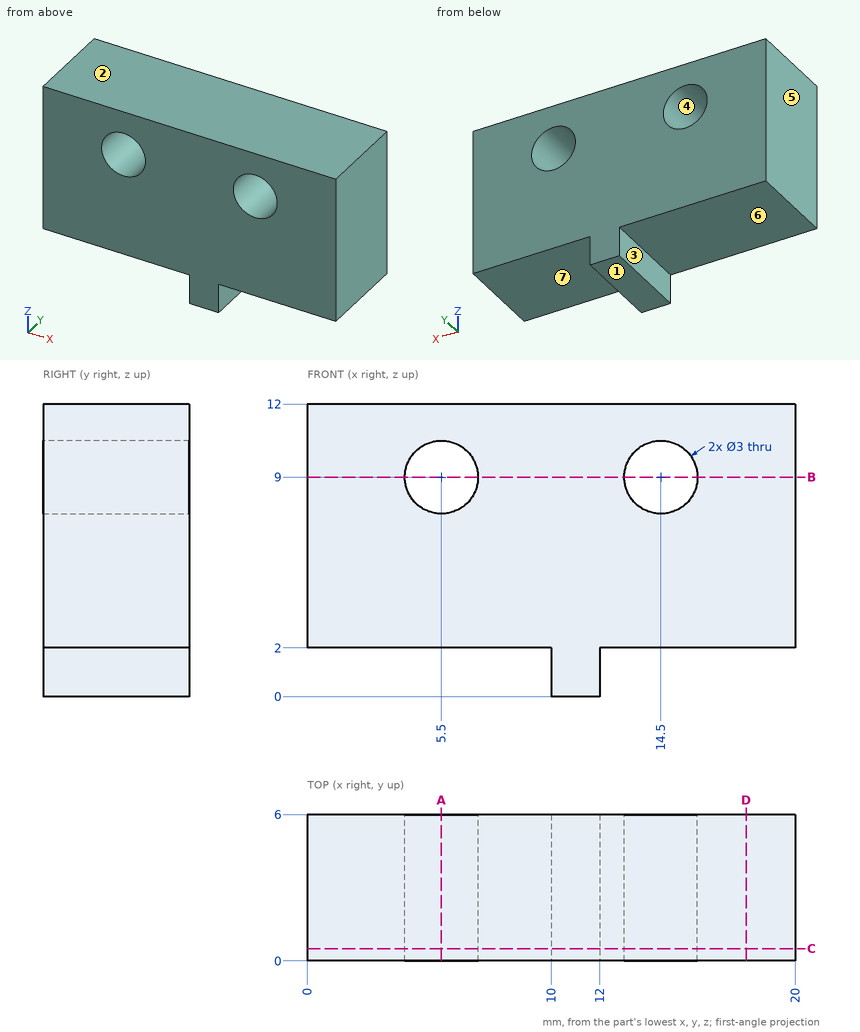
Answer from the drawing. Dimensions are ordinates in mm from the lowest x, y and z of the part. A direction names the side the tool comes from. Give positions to 0.01 mm unless a question says otherwise; leave off trailing zeros. Order: outer loops, then holes, each group sorted by start corner. A loop starts at its lowest first (then second) coordinate and runs counter-clockwise, first axis right, second up.
(1) Find section A-A (x = 5.5). Give the vertices of the cut face in (y, z).
(2) Straight lines are drawn through the part: L1, parallel to X at y = 4.35, z = 9; L2, parallel to Z at x = 5.5, y = 1.35; L3, parallel to X at y = 4.5, z = 10. For each, find the intervals that lie inside material, in ascending order.
(3) Given pin 1 (2 mm diameter, centred on y = 2.5, z = 0.5, fed in from +X); pin 2 (1.8 mm diameter, centred on x = 5, y = 4.5, fed in from -Z); pin 3 (0.6 mm diameter, centred on y = 2, z = 1, fed in from -X), each flat-ended and moving along its own axis, determine where each tip first touches the part or whether it passes through.
(4) For a pull along Z with two mould halves and no side action, classify the marked faces 1, 2, 3 and 4 as released by +Z, released by -Z, zero draft, split by the parting line, or undercut.
(5) Find section D-D (x = 18). Give the vertices of the cut face in (y, z).
(6) Find section B-B (z = 9). Give the vertices of the cut face in (x, y).
(7) Find section C-C (y = 0.5). Give the vertices of the cut face in (x, z).
(8) For the marked faces 5, 6 and 7, determine the directions among +Z, -Z, +X, -X, +Y, -Y from which every point of the face is accessible in a straight line to the end or side of a thin tool.
Result sheet:
1. outline: (0, 2) - (6, 2) - (6, 7.5) - (0, 7.5) - close; (0, 10.5) - (6, 10.5) - (6, 12) - (0, 12) - close
2. L1: x = 0 to 4, 7 to 13, 16 to 20
2. L2: z = 2 to 7.5, 10.5 to 12
2. L3: x = 0 to 4.38, 6.62 to 13.38, 15.62 to 20
3. pin 1: stops at x = 12
3. pin 2: stops at z = 2
3. pin 3: stops at x = 10
4. face 1: released by -Z
4. face 2: released by +Z
4. face 3: zero draft
4. face 4: undercut
5. outline: (0, 2) - (6, 2) - (6, 12) - (0, 12) - close
6. outline: (0, 0) - (4, 0) - (4, 6) - (0, 6) - close; (7, 0) - (13, 0) - (13, 6) - (7, 6) - close; (16, 0) - (20, 0) - (20, 6) - (16, 6) - close
7. outline: (0, 2) - (10, 2) - (10, 0) - (12, 0) - (12, 2) - (20, 2) - (20, 12) - (0, 12) - close; hole circle Ø3 at (5.5, 9); hole circle Ø3 at (14.5, 9)
8. face 5: +Z, -Z, -X, +Y, -Y
8. face 6: -Z, -X, +Y, -Y
8. face 7: -Z, +X, +Y, -Y
